Geometry: final body of the model. Coordinates: model frame, mm. A direction names the side the tool comes from. Give positions to 0.01 mm unless a question says otherwise; leave off trailing zeros. Loops run counter-clockwise (first coordinate to the right, second up) from the corner with the lowest first, then second, coordinate; pieces in that order, holes last. Notation, with made-up numbers: M -36.5,72 L -32.5,72 A14 ccw -32.5,83 Z; hole C -40,18.25 d8. An arc over 180 degrees is marked long. Put each result on its own line as item: value.
```python
from build123d import *

# Parameters (mm, degrees)
IZIM1_R                     = 1.6
Y_KSEKLIK_EKSTR_ZYON1_DEPTH = 4
IZIM3_R                     = 5.5
IZIM3_R_2                   = 1.6
Y_KSEKLIK_EKSTR_ZYON3_DEPTH = 3
KES_EKSTR_ZYON1_DEPTH       = 4


with BuildPart() as part:
    # Çizim1 → Yükseklik-Ekstrüzyon1 (new body)
    with BuildSketch(Plane.XY):
        with BuildLine():
            ThreePointArc((-5.273709113, -1.561407118), (3.018112795, -4.597933792), (3.530207231, 4.2175392))
            ThreePointArc((3.530207231, 4.2175392), (2, 17.25), (3.530207231, 30.2824608))
            ThreePointArc((3.530207231, 30.2824608), (3.018112795, 39.097933792), (-5.273709113, 36.061407118))
            ThreePointArc((-5.273709113, 36.061407118), (-8, 17.25), (-5.273709113, -1.561407118))
        make_face()
        with Locations((0, 34.5)):
            Circle(IZIM1_R, mode=Mode.SUBTRACT)
        Circle(IZIM1_R, mode=Mode.SUBTRACT)
    extrude(amount=Y_KSEKLIK_EKSTR_ZYON1_DEPTH)

    # Çizim3 → Yükseklik-Ekstrüzyon3 (add)
    with BuildSketch(Plane.XY.offset(4)):
        with Locations(Location((0, 34.5, 0), (0, 0, 163.507358371))):
            Circle(IZIM3_R)
        with Locations((0, 34.5)):
            Circle(IZIM3_R_2, mode=Mode.SUBTRACT)
    extrude(amount=Y_KSEKLIK_EKSTR_ZYON3_DEPTH)

    # Çizim4 → Kes-Ekstrüzyon1 (cut)
    with BuildSketch(Plane(origin=(0, 0, 0), x_dir=(-1, 0, 0), z_dir=(0, 0, -1))):
        Polygon((2.9, 36.174315781), (0, 37.848631561), (-2.9, 36.174315781), (-2.9, 32.825684219), (0, 31.151368439), (2.9, 32.825684219), align=None)
    extrude(amount=-KES_EKSTR_ZYON1_DEPTH, mode=Mode.SUBTRACT)


solid = part.part
```
Item 1: Set-up query: faces 1 (the flat face through (2.9, 35, 2)), 2 (the cylindrical face through (2.897, -4.675, 1.972)). Return all of +Z, -Z, +X, -X, +Y, -Y with unobstructed straight access to the full face (end or side cutting, diameter ignored); none if empty.
Output values:
face 1: -Z
face 2: +Z, -Z
Item 2: Section C-C on x = 1. Output: boundary loops of the cut face in (y, z), then the cut area to 3 significant figures.
Output values:
outline: M -5.41,0 L -1.25,0 L -1.25,4 L -5.41,4 Z; M 1.25,0 L 31.73,0 L 31.73,4 L 33.25,4 L 33.25,7 L 29.09,7 L 29.09,4 L 1.25,4 Z; M 35.75,4 L 37.27,4 L 37.27,0 L 39.91,0 L 39.91,7 L 35.75,7 Z
area: 174 mm²
Item 3: Mould query, pull axis X, two halves, no side actions, for faces 3 (the cylindrical face through (2, 17, 2)), 4 (the flat face through (1.43, 37.023, 1.972)), 5 (the flat face through (-1, 18, 0)). Classes: pulls with the +X half, pulls with the -X half, needs draft (parallel to the pull), parting line crosses it, or undercut.
Output values:
face 3: pulls with the +X half
face 4: undercut
face 5: needs draft
Item 4: Pin query (flat end, axial travel): pin 1 Ø1 at (x, y) = (-1.5, 24) entering from +Z; pin 2 Ø3.5 at (x, y) = (0, 34.5) entering from -Z; pin 3 Ø1 at (y, z) = (34, 2.5) entering from -X; pin 4 Ø3 at (y, z) = (20.5, 6) entering from -X. Return the tip coordinate at first contact, or that it passes through.
Output values:
pin 1: z = 4
pin 2: z = 4
pin 3: x = -5.98
pin 4: through
Item 5: Section B-B on y = 0. Output: boundary loops of the cut face in (x, z).
Output values:
outline: M -5.72,0 L -1.6,0 L -1.6,4 L -5.72,4 Z; M 1.6,0 L 5.5,0 L 5.5,4 L 1.6,4 Z
Item 6: Line query: probe 1 along Y at (x, z) = (0, 2.55); probe 2 along Y at (x, z) = (0, 4.9); probe 3 along Z at (x, y) = (4.5, 3). Output: solid intervals per line, ascending. Write a range as [from, to].
Output values:
probe 1: [-5.5, -1.6], [1.6, 31.15], [37.85, 40]
probe 2: [29, 32.9], [36.1, 40]
probe 3: [0, 4]
Item 7: Section A-A on z = 3. Count the separate pieces of the cut face and the enclosed holes in it, then the cut area to 3 significant figures.
Output values:
separate pieces: 1
enclosed holes: 2
area: 415 mm²
Item 8: Section D-D on z = 6. Output: boundary loops of the cut face in (x, y), then the cut area to 3 significant figures.
Output values:
outline: C 0,34.5 d11; hole C 0,34.5 d3.2
area: 87.0 mm²
